Part model, mm, in its own coordinate system. A direction names the side the tool comes from. Give positions to 0.01 mm unless a question says otherwise; leave off trailing zeros. Write each loop counter-clockwise with the first axis right and the second up, starting at its lowest first coordinate (ties: lowest second). Pieces come first, ordered by that corner, then holes.
```python
from build123d import *
from OCP.BRepFilletAPI import BRepFilletAPI_MakeChamfer

# Parameters (mm, degrees)
BOSS_EXTRUDE1_DEPTH = 20
FILLET1_R           = 2.5
SKETCH3_W           = 20
SKETCH3_H           = 5.625
SKETCH3_H_2         = 5.62
BOSS_EXTRUDE2_DEPTH = 16
FILLET2_R           = 10
SKETCH4_R           = 2.5
CUT_EXTRUDE1_DEPTH  = 74.488094444
SKETCH5_W           = 40
SKETCH5_H           = 5.62
BOSS_EXTRUDE3_DEPTH = 15
CHAMFER1_SIZE       = 35.337785487
CHAMFER1_SIZE_2     = 15
SKETCH6_R           = 2.5
CUT_EXTRUDE2_DEPTH  = 74.488094444
CUT_EXTRUDE3_DEPTH  = 10
BOSS_EXTRUDE4_DEPTH = 20
BOSS_EXTRUDE5_DEPTH = 20
BOSS_EXTRUDE6_DEPTH = 10
SKETCH12_R          = 2.5
CUT_EXTRUDE5_DEPTH  = 15


with BuildPart() as part:
    # Sketch1 → Boss-Extrude1 (new body)
    with BuildSketch(Plane(origin=(0, 0, 0), x_dir=(1, 0, 0), z_dir=(0, 1, 0))):
        with BuildLine():
            Line((40, -35), (-40, -35))
            ThreePointArc((-40, -35), (-47.071067812, -32.071067812), (-50, -25))
            Line((-50, -25), (-50, 25))
            ThreePointArc((-50, 25), (-47.071067812, 32.071067812), (-40, 35))
            Line((-40, 35), (40, 35))
            ThreePointArc((40, 35), (47.071067812, 32.071067812), (50, 25))
            Line((50, 25), (50, -25))
            ThreePointArc((50, -25), (47.071067812, -32.071067812), (40, -35))
        make_face()
    extrude(amount=BOSS_EXTRUDE1_DEPTH)

    # Fillet1
    fillet1_edges = [part.edges().sort_by_distance(p)[0] for p in [
        (-47.071067812, 20, 32.071067812),
        (0, 20, 35),
        (47.071067812, 20, 32.071067812),
        (50, 20, 0),
        (47.071067812, 20, -32.071067812),
        (0, 20, -35),
        (-47.071067812, 20, -32.071067812),
        (-50, 20, 0),
    ]]
    fillet(fillet1_edges, radius=FILLET1_R)

    # Sketch3 → Boss-Extrude2 (add)
    with BuildSketch(Plane.XZ):
        with Locations((-40, 4.0625)):
            Rectangle(SKETCH3_W, SKETCH3_H)
        with Locations((-40, 12.1925)):
            Rectangle(SKETCH3_W, SKETCH3_H)
        with Locations((-40, -12.1825)):
            Rectangle(SKETCH3_W, SKETCH3_H)
        with Locations((-40, -4.06)):
            Rectangle(SKETCH3_W, SKETCH3_H_2)
    extrude(amount=BOSS_EXTRUDE2_DEPTH)

    # Fillet2
    fillet2_edges = [part.edges().sort_by_distance(p)[0] for p in [
        (-30, -16, -12.1825),
        (-30, -16, -4.06),
        (-30, -16, 4.0625),
        (-30, -16, 12.1925),
        (-50, -16, -12.1825),
        (-50, -16, -4.06),
        (-50, -16, 4.0625),
        (-50, -16, 12.1925),
    ]]
    fillet(fillet2_edges, radius=FILLET2_R - 0.0001)  # a hair under: the kernel refuses the full size

    # Sketch4 → Cut-Extrude1 (cut, through all)
    with BuildSketch(Plane.XY.offset(15.005)):
        with Locations((-40, -8.5)):
            Circle(SKETCH4_R)
    extrude(amount=-CUT_EXTRUDE1_DEPTH, mode=Mode.SUBTRACT)

    # Sketch5 → Boss-Extrude3 (add)
    with BuildSketch(Plane.XZ):
        with Locations((-20, 4.06)):
            Rectangle(SKETCH5_W, SKETCH5_H)
        with Locations((-20, -4.06)):
            Rectangle(SKETCH5_W, SKETCH5_H)
    extrude(amount=BOSS_EXTRUDE3_DEPTH)

    # Chamfer1
    chamfer1_edges_1 = [part.edges().sort_by_distance(p)[0] for p in [
        (0, -15, -4.06),
    ]]
    chamfer1_side_1 = [part.faces().sort_by_distance(p)[0] for p in [
        (-0.3, -15, -4.06),
    ]]
    chamfer1_edges_2 = [part.edges().sort_by_distance(p)[0] for p in [
        (0, -15, 4.06),
    ]]
    chamfer1_side_2 = [part.faces().sort_by_distance(p)[0] for p in [
        (0, -14.7, 4.06),
    ]]
    chamfer1 = BRepFilletAPI_MakeChamfer(part.part.solid().wrapped)
    for e in chamfer1_edges_1:
        chamfer1.Add(CHAMFER1_SIZE - 0.0001, CHAMFER1_SIZE_2 - 0.0001, e.wrapped, chamfer1_side_1[0].wrapped)
    for e in chamfer1_edges_2:
        chamfer1.Add(CHAMFER1_SIZE_2 - 0.0001, CHAMFER1_SIZE - 0.0001, e.wrapped, chamfer1_side_2[0].wrapped)
    add(Compound.cast(chamfer1.Shape()), mode=Mode.REPLACE)  # a hair under: the kernel refuses the full size

    # Sketch6 → Cut-Extrude2 (cut, through all)
    with BuildSketch(Plane.XY.offset(15.005)):
        with Locations((-40, -8.5)):
            Circle(SKETCH6_R)
    extrude(amount=-CUT_EXTRUDE2_DEPTH, mode=Mode.SUBTRACT)

    # Sketch7 → Cut-Extrude3 (cut)
    with BuildSketch(Plane(origin=(0, 20, 0), x_dir=(1, 0, 0), z_dir=(0, 1, 0))):
        with BuildLine():
            Line((0, -33.5), (0, -42.5))
            Line((0, -42.5), (20, -42.5))
            Line((20, -42.5), (20, -33.5))
            ThreePointArc((20, -33.5), (20.292893219, -32.792893219), (21, -32.5))
            Line((21, -32.5), (39, -32.5))
            ThreePointArc((39, -32.5), (39.707106781, -32.207106781), (40, -31.5))
            Line((40, -31.5), (40, 32.5))
            Line((40, 32.5), (-20, 32.5))
            Line((-20, 32.5), (-20, -31.5))
            ThreePointArc((-20, -31.5), (-19.707106781, -32.207106781), (-19, -32.5))
            Line((-19, -32.5), (-1, -32.5))
            ThreePointArc((-1, -32.5), (-0.292893219, -32.792893219), (0, -33.5))
        make_face()
    extrude(amount=-CUT_EXTRUDE3_DEPTH, mode=Mode.SUBTRACT)

    # Sketch8 → Boss-Extrude4 (add)
    with BuildSketch(Plane(origin=(-20, 0, 0), x_dir=(0, 0, -1), z_dir=(1, 0, 0))):
        Polygon((32.5, 10), (27.5, 20), (32.5, 20), align=None)
    extrude(amount=BOSS_EXTRUDE4_DEPTH)

    # Sketch9 → Boss-Extrude5 (add)
    with BuildSketch(Plane.ZY.offset(-40)):
        Polygon((-32.5, 10), (-27.5, 20), (-32.5, 20), align=None)
    extrude(amount=BOSS_EXTRUDE5_DEPTH)

    # Sketch10 → Boss-Extrude6 (add)
    with BuildSketch(Plane.XZ):
        with BuildLine():
            Line((-5, 35), (25, 35))
            Line((25, 35), (18.449489743, 45.348469228))
            ThreePointArc((18.449489743, 45.348469228), (10, 50), (1.550510257, 45.348469228))
            Line((1.550510257, 45.348469228), (-5, 35))
        make_face()
    extrude(amount=-BOSS_EXTRUDE6_DEPTH)

    # Sketch12 → Cut-Extrude5 (cut)
    with BuildSketch(Plane(origin=(0, 10, 0), x_dir=(1, 0, 0), z_dir=(0, 1, 0))):
        with Locations(Location((10, -40, 0), (0, 0, 270))):
            Circle(SKETCH12_R)
    extrude(amount=-CUT_EXTRUDE5_DEPTH, mode=Mode.SUBTRACT)


solid = part.part
```
1) Saw through at D-D, the plane y = 12. Write the cut outline in (x, z), then the cut area to 3 significant figures.
Answers follow:
outline: (-50, -25) arc R10 ccw to (-40, -35) - (40, -35) arc R10 ccw to (50, -25) - (50, 25) arc R10 ccw to (40, 35) - (20, 35) - (20, 33.5) arc R1 ccw to (21, 32.5) - (39, 32.5) arc R1 cw to (40, 31.5) - (40, -31.5) - (20, -31.5) - (20, -32.5) - (0, -32.5) - (0, -31.5) - (-20, -31.5) - (-20, 31.5) arc R1 cw to (-19, 32.5) - (-1, 32.5) arc R1 ccw to (0, 33.5) - (0, 35) - (-40, 35) arc R10 ccw to (-50, 25) - close
area: 3,000 mm2
2) Saw through at B-B, the plane z = 23.5. Write the cut outline in (x, y).
Answers follow:
outline: (-50, 0) - (50, 0) - (50, 17.5) arc R2.5 ccw to (47.5, 20) - (40, 20) - (40, 10) - (-20, 10) - (-20, 20) - (-47.5, 20) arc R2.5 ccw to (-50, 17.5) - close
3) Saw through at A-A, the plane x = 10. Write the cut outline in (y, z).
Answers follow:
outline: (0, -35) - (17.5, -35) arc R2.5 ccw to (20, -32.5) - (10, -32.5) - (10, 37.5) - (0, 37.5) - close; (0, 42.5) - (10, 42.5) - (10, 50) - (0, 50) - close
4) Wall check: L1, parallel to Z at x = -31.5, y = -0.5 (3 decimals); L2, parallel to Z at x = -15.5, y = -6; L3, parallel to Y at x = -40, z = -4.5. Give the ranges that are in metal, low to high.
Answers follow:
L1: z = -14.995 to -9.37, -6.87 to -1.25, 1.25 to 6.875, 9.38 to 15.005
L2: z = -6.87 to -1.25, 1.25 to 6.87
L3: y = -16 to -11, -6 to 20
5) Saw through at C-C, the plane z = 40. Write the cut outline in (x, y).
Answers follow:
outline: (-1.84, 0) - (7.5, 0) - (7.5, 10) - (-1.84, 10) - close; (12.5, 0) - (21.84, 0) - (21.84, 10) - (12.5, 10) - close
6) Two-plate mould, pull along Z, no slides. Class faces 1 (the face through (29.86, 19.248, 34.287)), 2 (the face through (-30, -3, 12)), 3 (the face through (-10, 15, 32.5)): +Z half, -Z half, draft (parallel to the pull), parting line (faces both ways), or undercut.
Answers follow:
face 1: +Z half
face 2: draft
face 3: undercut
7) 3-axis set-ups, long thin cutter, end or side, ignore diameter. For faces 4 (the face through (47.15, 8.63, 31.99)), 5 (the face through (-32.85, -12.99, -12.14)), 6 (the face through (10, 15, -32.5)), 7 (the face through (-1, 9, -35)), 8 (the face through (-38, -6, -14.995)): which of +Z, -Z, +X, -X, +Y, -Y reach the whole face in a straight line?
Answers follow:
face 4: +Z, +X, +Y, -Y
face 5: -Z, +X, -Y
face 6: +Z, +Y
face 7: -Z, +X, -X, +Y, -Y
face 8: -Z, +X, -X, -Y
8) Pin check, flat tips, straight feed: pin 1 Ø8 at (x, y) = (-40, -8.5) entering from -Z (3 decimals); pin 2 Ø6 at (y, z) = (-2.5, -12.5) entering from +X; pin 3 Ø2 at (y, z) = (14, 30.5) entering from +X; pin 4 Ø4 at (y, z) = (12.5, -31) entering from -X. Stop position of each tip, or through.
Answers follow:
pin 1: stops at z = -14.995
pin 2: stops at x = 50
pin 3: stops at x = 48.93
pin 4: stops at x = -49.17
